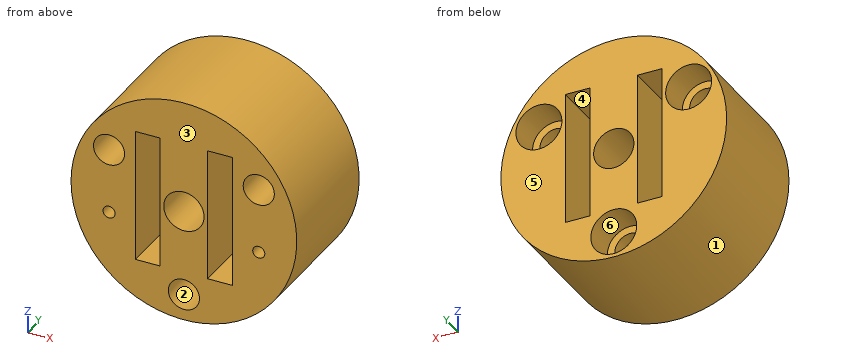
Autodesk Inventor part; units mm, degrees
ref_plane "YZ Plane" through (0, 0, 0) normal (1, 0, 0) x (0, 1, 0)
ref_plane "XZ Plane" through (0, 0, 0) normal (0, 1, 0) x (-1, 0, 0)
ref_plane "XY Plane" through (0, 0, 0) normal (0, 0, 1) x (1, 0, 0)
sketch "Sketch1" plane through (0, 0, 0) normal (0, 1, 0) x (-1, 0, 0)
  line L0 (0, 0) -> (13.6144, 0)
  circle A0 centre (0, 0) radius 17.78
  dimension "d0" = 13.6144
  dimension "d1" = 35.56
extrude "Extrusion1" add sketch "Sketch1" along normal blind 19.05
sketch "Sketch3" plane through (0, 19.05, 0) normal (0, 1, 0) x (1, 0, 0)
  line L0 (0, 0) -> (0, 13.6144)
  line L1 (0, 0) -> (13.6144, 0) construction
  dimension "d4" = 13.6144
  dimension "d5" = 90
hole "Hole1" at (0, 19.05, -13.6144) direction (0, -1, 0) diameter 4.9022 end through all counterbore diameter 7.239 counterbore depth 5.08
sketch "Sketch4" plane through (0, 0, 0) normal (0, -1, 0) x (1, 0, 0)
  circle A0 centre (0, -13.6144) radius 2.4511
  line L0 (0, 0) -> (0, -13.6144)
hole "Hole2" at (0, 0, -13.6144) direction (0, 1, 0) diameter 4.9022 depth 6.35
pattern_circular "Circular Pattern1" count 3 over 360 about axis through (0, 0, 0) along (0, 1, 0) of "Hole1", "Hole2"
sketch "Sketch6" plane through (0, 19.05, 0) normal (0, 1, 0) x (1, 0, 0)
  point P0 (0, 0)
  point P1 (0, 0)
hole "Hole3" at (0, 19.05, 0) direction (0, -1, 0) diameter 6.35 end through all
sketch "Sketch18" plane through (0, 0, 0) normal (0, -1, 0) x (1, 0, 0)
  circle A0 centre (-11.7904, 6.8072) radius 2.4511
  circle A1 centre (-11.7904, 6.8072) radius 4.1697
  circle A2 centre (0, 0) radius 3.7517
  line L0 (-7.6207, 6.8072) -> (-7.6207, -16.064)
  circle A3 centre (0, 0) radius 17.78
  line L1 (-7.6207, 6.8072) -> (-7.6207, 16.064)
  line L2 (-3.7517, 0) -> (-3.7517, -17.4687)
  line L3 (-3.7517, -17.4687) -> (-3.7517, 17.2429)
  circle A4 centre (11.7904, 6.8072) radius 2.4511
  circle A5 centre (11.7904, 6.8072) radius 4.1697
  line L4 (7.6207, 6.8072) -> (7.6207, -16.064)
  line L5 (7.6207, 16.064) -> (7.6207, 6.8072)
  line L6 (-7.6207, 10.9769) -> (-3.7517, 10.9769)
  line L7 (-6.9141, -9.9949) -> (-3.7517, -9.9949)
  line L8 (-7.6207, -9.9949) -> (-6.5754, -9.9949)
  line L9 (3.7517, 10.9769) -> (7.6207, 10.9769)
  line L10 (3.7517, -9.9949) -> (7.6207, -9.9949)
  line L11 (0, 0) -> (3.7517, 0)
  line L12 (3.7517, 0) -> (3.7517, 10.8227)
  line L13 (3.7517, 10.8227) -> (3.7517, -9.9949)
  line L14 (3.7517, 10.8227) -> (3.7517, 10.9769)
  line L15 (7.6207, 10.9769) -> (3.7517, 10.9769)
  point P0 (3.7517, 0)
extrude "Extrusion6" cut sketch "Sketch18" against normal blind 19.05 contours L1 L6 L3 L2 L7 L8 L0 | L5 L4 L10 L13 L12 L14 L9
sketch "Sketch21" plane through (0, 0, 0) normal (0, -1, 0) x (1, 0, 0)
  circle A0 centre (11.7904, 6.8072) radius 2.4511
  circle A1 centre (0, -13.6144) radius 2.4511
  line L0 (11.7904, 6.8072) -> (0, -13.6144)
  circle A2 centre (-11.7904, 6.8072) radius 2.4511
  line L1 (0, -13.6144) -> (-11.7904, 6.8072)
  line L2 (-11.7904, 6.8072) -> (11.7904, 6.8072)
  line L3 (11.7904, 6.8072) -> (11.7904, -13.6144)
  line L4 (11.7904, -13.6144) -> (0, -13.6144)
  line L5 (0, -13.6144) -> (-11.7904, -13.6144)
  line L6 (-11.7904, -13.6144) -> (-11.7904, 6.8072)
  circle A3 centre (11.7904, -3.4036) radius 0.635
  circle A4 centre (-11.7904, -3.4036) radius 0.635
  point P0 (0, 0)
  dimension "d68" = 1.27
hole "Hole6" at (-11.7904, 0, -3.4036) at (11.7904, 0, -3.4036) direction (0, 1, 0) diameter 1.905 depth 6.35
properties part number "table"
Part model, mm, in its own coordinate system. Face numbers are marked on the shaded views. A direction names the side the tool comes from. Coordinates: 2 decimals unless noted, no trailing zeros. Write each loop counter-clockwise with the first axis right and the second up, starting at its lowest first coordinate (ties: lowest second). Pieces come first, ordered by that corner, then holes. Notation, with made-up numbers: M 67,-27.75 L 102,-27.75 A10 cw 102,-15.75 Z; hole C -14.5,8 d5. An arc over 180 degrees is marked long. Return JSON: item names as keys, results as strings.
1. Pull direction Z, two halves, no side cores. Call the marked faces 1, 2 and 3: pulls with the +Z half, pulls with the -Z half, needs draft (parallel to the pull), parting line crosses it, or undercut.
Determined:
{"face 1": "parting line crosses it", "face 2": "undercut", "face 3": "needs draft"}
2. 3-axis set-ups, long thin cutter, end or side, ignore diameter. For the marked faces 4, 5 and 6: which of +Z, -Z, +X, -X, +Y, -Y reach the whole face in a straight line?
Determined:
{"face 4": "+Y, -Y", "face 5": "+Z, -Z, +X, -X, +Y", "face 6": "+Y"}
3. Saw through at B-B, the plane x = 0. Count the separate pieces of the cut face and the enclosed holes in it, then the cut area to 3 significant figures.
Determined:
{"separate pieces": "3", "enclosed holes": "0", "area": "451 mm²"}
4. Saw through at A-A, the plane z = 0. Write the cut outline in (x, y) (3 decimals), then the cut area to 3 significant figures.
Determined:
{"outline": "M -17.78,0 L -7.621,0 L -7.621,19.05 L -17.78,19.05 Z; M -3.752,0 L -3.175,0 L -3.175,19.05 L -3.752,19.05 Z; M 3.175,0 L 3.752,0 L 3.752,19.05 L 3.175,19.05 Z; M 7.621,0 L 17.78,0 L 17.78,19.05 L 7.621,19.05 Z", "area": "409 mm²"}
5. Flat gauge pins, fed straight in: pin 1 Ø1.7 at (x, z) = (-11.79, -3.4) entering from -Y; pin 2 Ø6.5 at (x, z) = (-11.79, 6.81) entering from +Y; pin 3 Ø5.5 at (x, z) = (0, 0) entering from +Y; pin 4 Ø1.2 at (x, y) = (6, 12.5) entering from +Z. Where does each tip first touch, or does it go through?
Determined:
{"pin 1": "y = 6.35", "pin 2": "y = 13.97", "pin 3": "through", "pin 4": "z = 16.94"}
6. Saw through at D-D, the plane z = -13. Write the cut outline in (x, y), then the cut area to 3 significant figures.
Determined:
{"outline": "M -12.13,0 L -2.37,0 L -2.37,13.97 L -3.57,13.97 L -3.57,19.05 L -12.13,19.05 Z; M 2.37,0 L 12.13,0 L 12.13,19.05 L 3.57,19.05 L 3.57,13.97 L 2.37,13.97 Z", "area": "360 mm²"}
7. Probe L1, parallel to Z at x = 0, y = 17.9 (3 decimals); L2, parallel to Z at x = 0, y = 3.25 (1 decimal); L3, parallel to X at y = 3, z = -9.5. List the from-to ranges inside material, lowest first.
Determined:
{"L1": "-17.78 to -17.234, -9.995 to -3.175, 3.175 to 17.78", "L2": "-17.8 to -16.1, -11.2 to -3.2, 3.2 to 17.8", "L3": "-15.03 to -7.62, -3.75 to 3.75, 7.62 to 15.03"}
